Geometry: final body of the model. Coordinates: model frame, mm. Give positions to 0.01 mm unless a question says otherwise; leave off trailing zeros. Order: outer loops, then holes, each group sorted by start corner. A loop starts at its lowest first (then second) coordinate and runs counter-clockwise, first axis right, second up. Notation, with made-up numbers: M 6,32 L 16,32 A16 ccw 16,55 Z; hole C 12.25,21 d6. An arc over 180 degrees is marked long. One line per item, written item: value. Start each with the question number.
```python
from build123d import *

# Parameters (mm, degrees)
BOSS_EXTRUDE1_DEPTH = 2


with BuildPart() as part:
    # Sketch1 → Boss-Extrude1 (new body)
    with BuildSketch(Plane(origin=(0, 0, 0), x_dir=(1, 0, 0), z_dir=(0, 1, 0))):
        with BuildLine():
            Line((-65.26908877, -1.246266978), (-65.26908877, -3.246266978))
            Line((-65.26908877, -3.246266978), (-40.019014758, -3.246266978))
            ThreePointArc((-40.019014758, -3.246266978), (-38.315467936, -10.540153027), (-41.26908877, -17.423391323))
            ThreePointArc((-41.26908877, -17.423391323), (-41.183302332, -20.160480541), (-38.446213114, -20.246266978))
            ThreePointArc((-38.446213114, -20.246266978), (-31.562974818, -17.292646145), (-24.26908877, -18.996192966))
            Line((-24.26908877, -18.996192966), (-24.26908877, -44.246266978))
            Line((-24.26908877, -44.246266978), (-22.26908877, -44.246266978))
            Line((-22.26908877, -44.246266978), (-22.26908877, -18.996192966))
            ThreePointArc((-22.26908877, -18.996192966), (-14.975202721, -17.292646145), (-8.091964425, -20.246266978))
            ThreePointArc((-8.091964425, -20.246266978), (-5.354875207, -20.160480541), (-5.26908877, -17.423391323))
            ThreePointArc((-5.26908877, -17.423391323), (-8.222709603, -10.540153027), (-6.519162781, -3.246266978))
            Line((-6.519162781, -3.246266978), (18.73091123, -3.246266978))
            Line((18.73091123, -3.246266978), (18.73091123, -1.246266978))
            Line((18.73091123, -1.246266978), (-6.519162781, -1.246266978))
            ThreePointArc((-6.519162781, -1.246266978), (-8.222709603, 6.04761907), (-5.26908877, 12.930857366))
            ThreePointArc((-5.26908877, 12.930857366), (-5.354875207, 15.667946584), (-8.091964425, 15.753733022))
            ThreePointArc((-8.091964425, 15.753733022), (-14.975202721, 12.800112188), (-22.26908877, 14.50365901))
            Line((-22.26908877, 14.50365901), (-22.26908877, 39.753733022))
            Line((-22.26908877, 39.753733022), (-24.26908877, 39.753733022))
            Line((-24.26908877, 39.753733022), (-24.26908877, 14.50365901))
            ThreePointArc((-24.26908877, 14.50365901), (-31.562974818, 12.800112188), (-38.446213114, 15.753733022))
            ThreePointArc((-38.446213114, 15.753733022), (-41.183302332, 15.667946584), (-41.26908877, 12.930857366))
            ThreePointArc((-41.26908877, 12.930857366), (-38.315467936, 6.04761907), (-40.019014758, -1.246266978))
            Line((-40.019014758, -1.246266978), (-65.26908877, -1.246266978))
        make_face()
    extrude(amount=BOSS_EXTRUDE1_DEPTH)


solid = part.part
```
Q1. Ray query, line 1 along X through (y, z) = (0.6, 40); line 2 along Z through (x, y) = (-43, 1.5); line 3 along Z through (x, y) = (-16.5, 1.8). Return the intervals inside material, ascending. Write a range as [from, to].
Q2. Contact query for flat-ended pins moving along their axis: pin 1 (1 mm diameter, centred on x = -53.5, y = 1, fed in from +Z); pin 2 (0.6 mm diameter, centred on y = 1.5, z = -29.5, fed in from +X); pin 3 (8 mm diameter, centred on x = -14.5, z = 26, fed in from -Y); pin 4 (1 mm diameter, centred on x = -58.5, y = 1.5, fed in from -Z). Output: stop coordinate, or through.
Q3. Section query B-B on z = -21. Return loops of the section in (x, y), and give its area (3 significant figures).
Q4. Mould query, pull axis Z, two halves, no side actions, for faces 1 (the face through (-22.269, 1, 32)), 2 (the face through (-23, 1, 44.246)), 3 (the face through (-41.15, 0.99, -15.7)). Classes: +Z half, -Z half, draft (parallel to the pull), parting line (faces both ways), or undercut.
Q5. Section query C-C on x = -59. Return loops of the section in (y, z), and give its area (3 significant figures).
Q6. Section query A-A on y = 0.3. Return loops of the section in (x, z), and give its area (3 significant figures).
Results below:
1. line 1: [-24.27, -22.27]
1. line 2: [1.25, 3.25]
1. line 3: [-12.76, 17.26]
2. pin 1: z = 3.25
2. pin 2: x = -22.27
2. pin 3: through
2. pin 4: z = 1.25
3. outline: M -24.27,0 L -22.27,0 L -22.27,2 L -24.27,2 Z
3. area: 4.00 mm2
4. face 1: draft
4. face 2: +Z half
4. face 3: undercut
5. outline: M 0,1.25 L 2,1.25 L 2,3.25 L 0,3.25 Z
5. area: 4.00 mm2
6. outline: M -65.27,1.25 L -40.02,1.25 A12 cw -41.27,-12.93 A2 ccw -38.45,-15.75 A12 cw -24.27,-14.5 L -24.27,-39.75 L -22.27,-39.75 L -22.27,-14.5 A12 cw -8.09,-15.75 A2 ccw -5.27,-12.93 A12 cw -6.52,1.25 L 18.73,1.25 L 18.73,3.25 L -6.52,3.25 A12 cw -5.27,17.42 A2 ccw -8.09,20.25 A12 cw -22.27,19 L -22.27,44.25 L -24.27,44.25 L -24.27,19 A12 cw -38.45,20.25 A2 ccw -41.27,17.42 A12 cw -40.02,3.25 L -65.27,3.25 Z
6. area: 1,240 mm2
